```python
from build123d import *

# Parameters (mm, degrees)
SKETCH006_W     = 70.5
SKETCH006_H     = 25.7
PAD003_DEPTH    = 9.5
THICKNESS001_T  = 2.5
SKETCH007_R     = 3
POCKET002_DEPTH = 75.501
SKETCH046_W     = 70.5
SKETCH046_H     = 1.5
PAD039_DEPTH    = 2.5
PAD002_DEPTH    = 2.5


with BuildPart() as body002:
    # Sketch006 → Pad003 (new body)
    with BuildSketch(Plane.XY):
        with Locations((0, -48)):
            Rectangle(SKETCH006_W, SKETCH006_H)
    extrude(amount=PAD003_DEPTH)

    # Thickness001
    thickness001_openings = [body002.faces().sort_by_distance(p)[0] for p in [
        (0, -48, 9.5),
        (0, -48, 0),
    ]]
    offset(amount=THICKNESS001_T, openings=thickness001_openings, kind=Kind.INTERSECTION)

    # Sketch007 (on Face6 of Thickness001) → Pocket002 (cut, through all)
    with BuildSketch(Plane(origin=(-37.75, 0, 0), x_dir=(0, -1, 0), z_dir=(-1, 0, 0))):
        with Locations((39, 4.75)):
            Circle(SKETCH007_R)
    extrude(amount=-POCKET002_DEPTH, mode=Mode.SUBTRACT)

    # Sketch046 → Pad039 (join)
    with BuildSketch(Plane.XY):
        with Locations((0, -35.75)):
            Rectangle(SKETCH046_W, SKETCH046_H)
    extrude(amount=PAD039_DEPTH)


with BuildPart() as body002_1:
    # Body002 placement: moved
    add(body002.part.moved(Location((84.5, 36.85, 0))))


with BuildPart() as middle:
    # Sketch005 → Pad002 (new body)
    with BuildSketch(Plane(origin=(0, 0, 0), x_dir=(1, 0, 0), z_dir=(0, 0, -1))):
        Polygon((-40.25, 30.15), (40.25, 30.15), (44.25, 30.15), (44.25, 36.5), (40.251921, 34.191708), (40.251921, 44.936467), (44.25, 42.628175), (44.25, 53.372934), (40.251921, 51.064642), (40.251921, 61.809401), (44.251921, 59.5), (44.251921, 65.85), (40.251921, 65.85), (-40.248079, 65.85), (-40.248079, 59.35), (-44.098079, 61.572799), (-44.098079, 51.293867), (-40.248079, 53.516665), (-40.248079, 42.486665), (-44.1, 44.706133), (-44.1, 34.427201), (-40.25, 36.65), align=None)
    extrude(amount=PAD002_DEPTH)


with BuildPart() as middle_1:
    # Body001 placement: moved
    add(middle.part.moved(Location((84.5, 36.85, 0))))

    # Fusion003: union Body002
    add(body002_1.part)


solid = middle_1.part
```
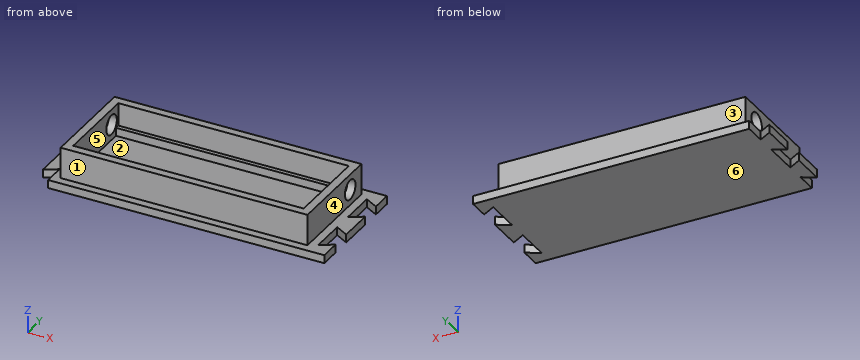
Build history of the part. All positions in model axes, mm. Face numbers are marked on the shaded views. A direction names the side the tool comes from. Give positions to 0.01 mm unless a question says otherwise; leave off trailing zeros. Loops run counter-clockwise (first coordinate to the right, second up) from the corner with the lowest first, then second, coordinate; pieces in that order, holes last.
1) 3-axis set-ups, long thin cutter, end or side, ignore diameter. For the marked faces 4, 5 and 6: which of +Z, -Z, +X, -X, +Y, -Y reach the whole face in a straight line?
Values follow:
face 4: +Z, +X, +Y, -Y
face 5: +Z
face 6: -Z, +X, -X, +Y, -Y
2) Two-plate mould, pull along Y, no slides. Class the marked faces 1, 2 and 3: released by +Y, released by -Y, zero draft, split by the parting line, or undercut.
Values follow:
face 1: released by -Y
face 2: undercut
face 3: released by +Y
3) Probe line 1 along Z through (x, y) = (48.15, -2.15); line 2 along X through (y, z) = (-21, 2.5); line 3 along Y through (x, z) = (112, 8.75). List the from-to ranges inside material, lowest first.
Values follow:
line 1: z = -2.5 to 1.75, 7.75 to 9.5
line 2: x = 46.75 to 49.25, 119.75 to 122.25
line 3: y = -26.5 to -24, 1.7 to 4.2
4) Drop flat-ended pins along their axis: P1, Ø5.5, axis at x = 79.5, z = 5, coming from the -Y side; P2, Ø5, axis at x = 57.5, y = -13.5, coming from the +Z side; P3, Ø0.8, axis at y = -25.5, z = -1.5, coming from the -X side; P4, Ø3.5, axis at y = -2.15, z = 4.75, coming from the -X side. Give the stop position or say it passes through.
Values follow:
P1: stops at y = -26.5
P2: stops at z = 0
P3: stops at x = 44.25
P4: passes through
5) Band-saw the part on B-B on y = -2. List the corners of the cut face in (x, z), then the cut area to 3 significant figures.
Values follow:
outline: (40.4, -2.5) - (124.75, -2.5) - (124.75, 0) - (122.25, 0) - (122.25, 1.75) - (119.75, 1.75) - (119.75, 0) - (49.25, 0) - (49.25, 1.75) - (46.75, 1.75) - (46.75, 0) - (40.4, 0) - close; (46.75, 7.75) - (49.25, 7.75) - (49.25, 9.5) - (46.75, 9.5) - close; (119.75, 7.75) - (122.25, 7.75) - (122.25, 9.5) - (119.75, 9.5) - close
area: 228 mm2
6) Band-saw the part on C-C on x = 89.5. List the corners of the cut face in (y, z), then the cut area to 3 significant figures.
Values follow:
outline: (-29, -2.5) - (6.7, -2.5) - (6.7, 0) - (4.2, 0) - (4.2, 9.5) - (1.7, 9.5) - (1.7, 2.5) - (0.35, 2.5) - (0.35, 0) - (-24, 0) - (-24, 9.5) - (-26.5, 9.5) - (-26.5, 0) - (-29, 0) - close
area: 140 mm2
7) Band-saw the part on A-A on z = 4.75. List the corners of the cut face in (x, y), then the cut area to 3 significant figures.
Values follow:
outline: (46.75, -26.5) - (122.25, -26.5) - (122.25, -5.15) - (119.75, -5.15) - (119.75, -24) - (49.25, -24) - (49.25, -5.15) - (46.75, -5.15) - close; (46.75, 0.85) - (49.25, 0.85) - (49.25, 1.7) - (119.75, 1.7) - (119.75, 0.85) - (122.25, 0.85) - (122.25, 4.2) - (46.75, 4.2) - close
area: 476 mm2
